Geometry: final body of the model. Coordinates: model frame, mm. A direction names the side the tool comes from. Round coordinates to 2 decimals unless told otherwise and drop trailing zeros. Loops run counter-clockwise (first coordinate to the right, second up) from the corner with the lowest first, then second, coordinate; pieces in that order, holes last. Notation, with made-up numbers: (40.25, -15) - (56.25, -15) arc R24 ccw to (56.25, 9) - close; hole circle Ø2 at (49.5, 81). An arc over 180 degrees is marked (long way). Answer as a JSON object with one key per item and string values. Group by question number.
Item 1: Section B-B (z = 12.5). Return the cut outline in (x, y), plus the area to 3 significant figures.
Item 2: First-contact query: pin 1 (7.5 mm diameter, centred on x = -16, z = 18, fed in from +Y); pin 2 (6 mm diameter, centred on x = -16.5, z = 22, fed in from -Y). Flat tips, straight axial feed; report the tip coordinate or a pass-through.
Item 3: Line query: line 1 (Y direction, x = -32, z = 18); line 2 (Z direction, x = -38, y = -13.5); line 3 (Z direction, x = -12, y = -6). Output: solid intervals per line, ascending.
Item 4: Section C-C (y = 4). Return the cut outline in (x, z), plus the area to 3 significant figures.
Item 5: Section A-A (x = -34). Return the cut outline in (y, z).
Item 6: Section D-D (y = -1). Return the cut outline in (x, z), plus the area to 3 significant figures.
Item 7: Reachability of faces 1 (the face through (-19, 0, 13)), 2 (the face through (-19, -12.7, 13)), 3 (the face through (-35, -7, 0)) from +Z, -Z, +X, -X, +Y, -Y: full face, straight path, thin tool, end or side. Return the list, or none.
```python
from build123d import *

# Parameters (mm, degrees)
F0_W      = 57.15
F0_H      = 25.4
F1_DEPTH  = 12.7
F2_W      = 31.75
F2_H      = 25.4
F3_DEPTH  = 12.7
F4_W      = 31.75
F4_H      = 25.4
F5_DEPTH  = 12.7
F7_DEPTH  = 12.7
F9_DEPTH  = 12.7
F11_DEPTH = 12.7


with BuildPart() as f1:
    # F0 (on Front) → F1 (new body)
    with BuildSketch(Plane.XZ):
        with Locations((-28.575, 12.7)):
            Rectangle(F0_W, F0_H)
    extrude(amount=F1_DEPTH)

    # F2 (on face) → F3 (join)
    with BuildSketch(Plane.XZ.offset(12.7)):
        with Locations((-41.275, 12.7)):
            Rectangle(F2_W, F2_H)
    extrude(amount=F3_DEPTH)

    # F4 (on face) → F5 (join)
    with BuildSketch(Plane(origin=(0, 0, 0), x_dir=(-1, 0, 0), z_dir=(0, 1, 0))):
        with Locations((41.275, 12.7)):
            Rectangle(F4_W, F4_H)
    extrude(amount=F5_DEPTH)

    # F6 (on face) → F7 (cut)
    with BuildSketch(Plane(origin=(0, 12.7, 0), x_dir=(-1, 0, 0), z_dir=(0, 1, 0))):
        Polygon((25.4, 25.4), (25.4, 0), (38.1, 25.4), align=None)
    extrude(amount=-F7_DEPTH, mode=Mode.SUBTRACT)

    # F8 (on face) → F9 (cut)
    with BuildSketch(Plane(origin=(0, 0, 0), x_dir=(-1, 0, 0), z_dir=(0, 1, 0))):
        Polygon((0, 25.4), (0, 0), (12.7, 25.4), align=None)
    extrude(amount=-F9_DEPTH, mode=Mode.SUBTRACT)

    # F10 (on face) → F11 (cut)
    with BuildSketch(Plane.XZ.offset(25.4)):
        Polygon((-38.1, 25.4), (-25.4, 0), (-25.4, 25.4), align=None)
    extrude(amount=-F11_DEPTH, mode=Mode.SUBTRACT)


solid = f1.part
```
Values:
{
 "1": {"outline": "(-57.15, -25.4) - (-31.65, -25.4) - (-31.65, -12.7) - (-6.25, -12.7) - (-6.25, 0) - (-31.65, 0) - (-31.65, 12.7) - (-57.15, 12.7) - close", "area": "1,290 mm^2"},
 "2": {"pin 1": "stops at y = 0", "pin 2": "stops at y = -12.7"},
 "3": {"line 1": "y = -12.7 to 0", "line 2": "z = 0 to 25.2", "line 3": "z = 0 to 24"},
 "4": {"outline": "(-57.15, 0) - (-25.4, 0) - (-38.1, 25.4) - (-57.15, 25.4) - close", "area": "645 mm^2"},
 "5": {"outline": "(-25.4, 0) - (12.7, 0) - (12.7, 17.2) - (0, 17.2) - (0, 25.4) - (-12.7, 25.4) - (-12.7, 17.2) - (-25.4, 17.2) - close"},
 "6": {"outline": "(-57.15, 0) - (0, 0) - (-12.7, 25.4) - (-57.15, 25.4) - close", "area": "1,290 mm^2"},
 "7": {"face 1": "+Z, +X, +Y", "face 2": "+Z, +X, -Y", "face 3": "-Z, +X, -X, +Y, -Y"}
}
